Can you work these out from the drawing? Everything is in mm from the part's minimum corner. A direction names the side the tool comes from. Give positions to 0.01 mm unless a question says otherwise; leave off trailing zeros. Write each loop counter-clockwise with the first axis right and the second up, starting at its lowest first coordinate (ties: lowest second). Pieces come first, ordered by that corner, then holes. Notation, with made-up numbers: (66, 52) - (88, 52) arc R20 ccw to (88, 58) - close; hole circle Ø11 at (-26.75, 24.5). An arc over 180 degrees is marked (long way). Use a Markdown table: item, result.
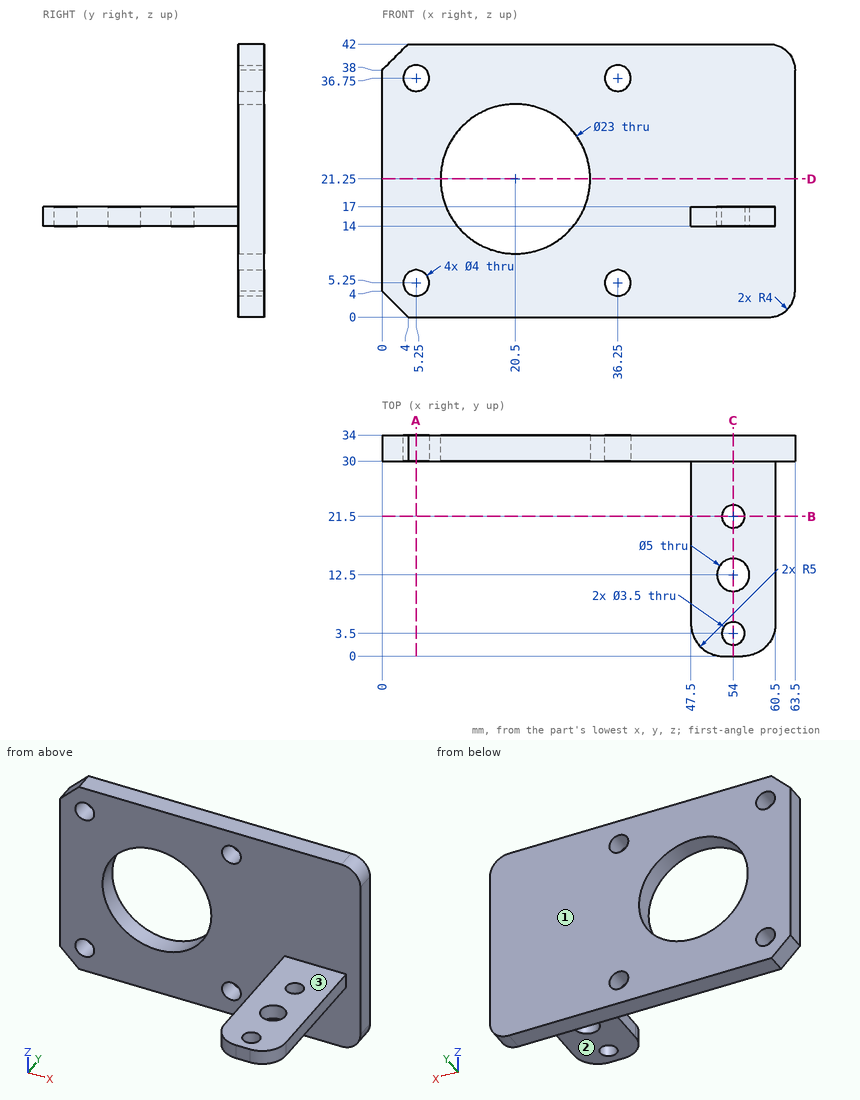
Item 1: If we section it at D-D, the plane z = 21.25: Write out the boundary of the cut face in (x, y), plus the area to 3 significant figures.
Values:
| item | result |
|---|---|
| outline | (0, 30) - (9, 30) - (9, 34) - (0, 34) - close; (32, 30) - (63.5, 30) - (63.5, 34) - (32, 34) - close |
| area | 162 mm2 |
Item 2: Will these pins go through, and if not, where does the flat tip stop? pin 1 Ø12 at (y, z) = (9.5, 6.5) entering from +X; pin 2 Ø5.5 at (x, y) = (54, 21.5) entering from -Z; pin 3 Ø12.5 at (x, z) = (18.5, 10.5) entering from -Y; pin 4 Ø4 at (x, y) = (51, 18.5) entering from +Z.
Values:
| item | result |
|---|---|
| pin 1 | passes through |
| pin 2 | stops at z = 14 |
| pin 3 | stops at y = 30 |
| pin 4 | stops at z = 17 |
Item 3: If we section it at A-A, the plane x = 5.25: Write out the boundary of the cut face in (y, z), plus the area to 3 significant figures.
Values:
| item | result |
|---|---|
| outline | (30, 0) - (34, 0) - (34, 3.25) - (30, 3.25) - close; (30, 7.25) - (34, 7.25) - (34, 34.75) - (30, 34.75) - close; (30, 38.75) - (34, 38.75) - (34, 42) - (30, 42) - close |
| area | 136 mm2 |
Item 4: If we section it at B-B, the plane y = 21.5: Write out the boundary of the cut face in (x, z).
Values:
| item | result |
|---|---|
| outline | (47.5, 14) - (52.25, 14) - (52.25, 17) - (47.5, 17) - close; (55.75, 14) - (60.5, 14) - (60.5, 17) - (55.75, 17) - close |
Item 5: For the marked faces 1, 2 and 3, which set-ups out of +Z, -Z, +X, -X, +Y, -Y let a thin tool reach every point of the face, with its end or its side?
Values:
| item | result |
|---|---|
| face 1 | +Z, -Z, +X, -X, +Y |
| face 2 | -Z, +X, -X, -Y |
| face 3 | +Z, +X, -X, -Y |
Item 6: I need wall thicknesses on line 1 along Z through (x, y) = (5, 31); line 2 along Y through (x, z) = (54, 16); line 3 along Z through (x, y) = (55, 6). Which ranges of each line are inside material? Lowest first, please. Write a range as [from, to].
Values:
| item | result |
|---|---|
| line 1 | z = [0, 3.27], [7.23, 34.77], [38.73, 42] |
| line 2 | y = [0, 1.75], [5.25, 10], [15, 19.75], [23.25, 34] |
| line 3 | z = [14, 17] |
Item 7: If we section it at C-C, the plane x = 54: Write out the boundary of the cut face in (y, z).
Values:
| item | result |
|---|---|
| outline | (0, 14) - (1.75, 14) - (1.75, 17) - (0, 17) - close; (5.25, 14) - (10, 14) - (10, 17) - (5.25, 17) - close; (15, 14) - (19.75, 14) - (19.75, 17) - (15, 17) - close; (23.25, 14) - (30, 14) - (30, 0) - (34, 0) - (34, 42) - (30, 42) - (30, 17) - (23.25, 17) - close |
